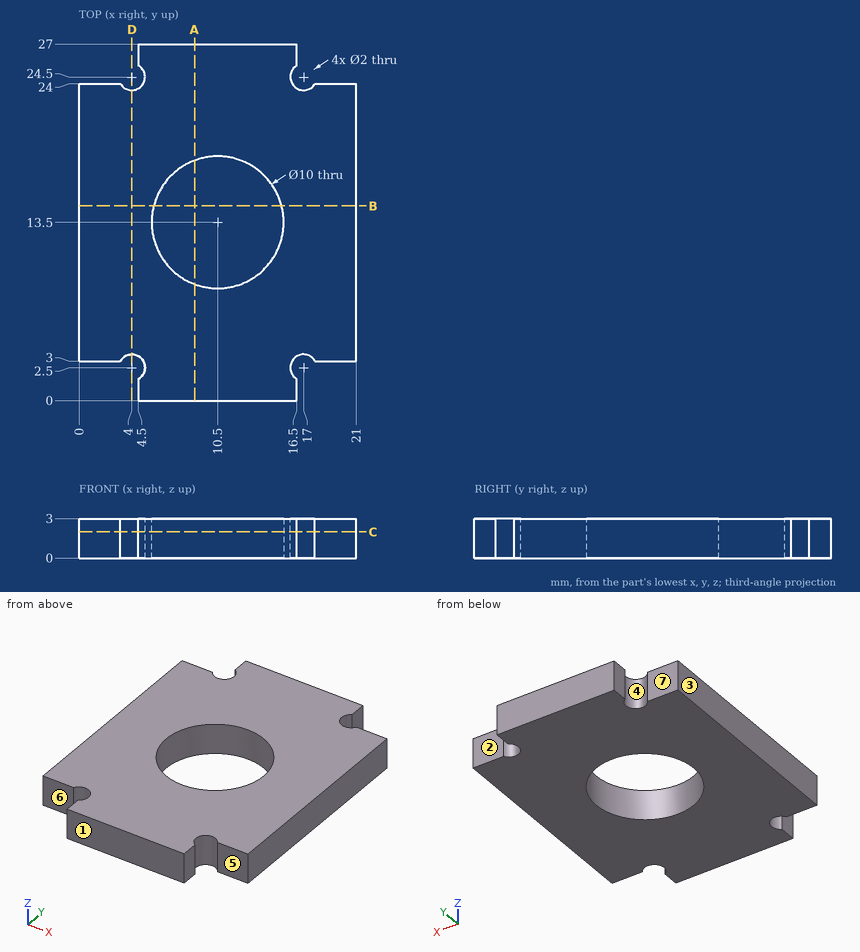
Study the drawing (mm; zero at the part's minimum x, y, z) and answer. A direction names the side the tool comes from. Coordinates: 2 decimals unless noted, no trailing zeros. Loops run counter-clockwise (first coordinate to the right, second up) from the corner with the lowest first, then second, coordinate; pieces in that order, holes last. Notation, with made-up numbers: (65, 3.25) -> (117, 3.25) arc R26 cw to (117, 30.25) -> close; hole circle Ø4 at (84.5, -26.75). An arc over 180 degrees is marked (long way). Write item = value, one per line. Start each with the question number.
1) For the marked faces 5, 6 and 7, determine the directions among +Z, -Z, +X, -X, +Y, -Y from which every point of the face is accessible in a straight line to the end or side of a thin tool.
2) The part is cut by section C-C, the plane z = 2. Determine the outline of the cut face in (x, y), plus the area to 3 significant figures.
3) The part is cut by section B-B, the plane y = 14.75. Determine the outline of the cut face in (x, z).
4) The mould has two halves that part along Y. Classify the marked faces 1, 2, 3 and 4: pulls with the +Y half, pulls with the -Y half, needs draft (parallel to the pull), parting line crosses it, or undercut.
5) Find the intervals of material crossed by L1, parallel to X at y = 24.5, z = 1.7; L2, parallel to Y at x = 17, z = 0.9; L3, parallel to Y at x = 2.5, z = 1.4, in increasing order. Write a range as from..to.
6) The part is cut by section A-A, the plane x = 8.75. Determine the outline of the cut face in (y, z), plus the area to 3 significant figures.
7) The part is cut by section D-D, the plane x = 4. Determine the outline of the cut face in (y, z).
8) Given P1, Ø11.5, axis at x = 10.5, y = 13.5, coming from the +Z side; P2, Ø0.8, axis at y = 26, z = 1, coming from the +X side; P3, Ø1.3, axis at y = 26, z = 1, coming from the -X side; P4, Ø0.9, axis at x = 1, z = 2, coming from the -Y side, each flat-ended and moving along its own axis, determine where each tip first touches the part or whether it passes through.
Result:
q1.face_5 = +Z, -Z, +X, -Y
q1.face_6 = +Z, -Z, -X, -Y
q1.face_7 = +Z, -Z, -X, +Y
q2.outline = (0, 3) -> (3.13, 3) arc R1 cw (long way) to (4.5, 1.63) -> (4.5, 0) -> (16.5, 0) -> (16.5, 1.63) arc R1 cw (long way) to (17.87, 3) -> (21, 3) -> (21, 24) -> (17.87, 24) arc R1 cw (long way) to (16.5, 25.37) -> (16.5, 27) -> (4.5, 27) -> (4.5, 25.37) arc R1 cw (long way) to (3.13, 24) -> (0, 24) -> close; hole circle Ø10 at (10.5, 13.5)
q2.area = 430 mm²
q3.outline = (0, 0) -> (5.66, 0) -> (5.66, 3) -> (0, 3) -> close; (15.34, 0) -> (21, 0) -> (21, 3) -> (15.34, 3) -> close
q4.face_1 = pulls with the -Y half
q4.face_2 = pulls with the +Y half
q4.face_3 = needs draft
q4.face_4 = undercut
q5.L1 = 5..16
q5.L2 = 3.5..23.5
q5.L3 = 3..24
q6.outline = (0, 0) -> (8.82, 0) -> (8.82, 3) -> (0, 3) -> close; (18.18, 0) -> (27, 0) -> (27, 3) -> (18.18, 3) -> close
q6.area = 52.9 mm²
q7.outline = (3.5, 0) -> (23.5, 0) -> (23.5, 3) -> (3.5, 3) -> close
q8.P1 = 3
q8.P2 = 16.5
q8.P3 = 4.5
q8.P4 = 3
